Check sheet for the modelled part. Datum: model origin and axes. Units: mm. Face numbers are marked on the shaded views. A direction names the side the tool comes from. Give positions to 0.01 mm unless a question says otherwise; leave off trailing zeros. Order: outer loops, then holes, each group sorted by start corner. A loop starts at its lowest first (then second) coordinate and runs counter-clockwise, first axis right, second up.
from build123d import *

# Parameters (mm, degrees)
SKETCH1_W           = 254
SKETCH1_H           = 63.5
BOSS_EXTRUDE1_DEPTH = 76.2
SHELL1_T            = -3.175
CUT_EXTRUDE1_REACH  = 163.145
SKETCH2_W           = 38.1
SKETCH2_H           = 25.4
SKETCH3_R           = 2.5
CUT_EXTRUDE2_DEPTH  = 162.144934764
SKETCH4_W           = 161.29
SKETCH4_H           = 40.64
CUT_EXTRUDE3_DEPTH  = 152.471127612


with BuildPart() as part:
    # Sketch1 → Boss-Extrude1 (new body)
    with BuildSketch(Plane(origin=(0, 0, 0), x_dir=(1, 0, 0), z_dir=(0, 1, 0))):
        Rectangle(SKETCH1_W, SKETCH1_H)
    extrude(amount=BOSS_EXTRUDE1_DEPTH)

    # Shell1
    shell1_openings = [part.faces().sort_by_distance(p)[0] for p in [
        (0, 0, 0),
    ]]
    offset(amount=SHELL1_T, openings=shell1_openings, kind=Kind.INTERSECTION)

    # Sketch2 → Cut-Extrude1 (cut, up to next)
    with BuildSketch(Plane.XY.offset(31.75), mode=Mode.PRIVATE) as cut_extrude1_sk1:
        with Locations((63.5, 38.1)):
            Rectangle(SKETCH2_W, SKETCH2_H)
    cut_extrude1_tool1 = extrude(cut_extrude1_sk1.sketch, amount=-CUT_EXTRUDE1_REACH, mode=Mode.PRIVATE) & part.part
    # Sketch2 → Cut-Extrude1 (cut, up to next)
    with BuildSketch(Plane.XY.offset(31.75), mode=Mode.PRIVATE) as cut_extrude1_sk2:
        with Locations((-63.5, 38.1)):
            Rectangle(SKETCH2_W, SKETCH2_H)
    cut_extrude1_tool2 = extrude(cut_extrude1_sk2.sketch, amount=-CUT_EXTRUDE1_REACH, mode=Mode.PRIVATE) & part.part
    add(cut_extrude1_tool1.solids().sort_by_distance((63.5, 38.1, 31.75))[0], mode=Mode.SUBTRACT)
    add(cut_extrude1_tool2.solids().sort_by_distance((-63.5, 38.1, 31.75))[0], mode=Mode.SUBTRACT)

    # Sketch3 → Cut-Extrude2 (cut, through all)
    with BuildSketch(Plane(origin=(0, 0, -31.75), x_dir=(-1, 0, 0), z_dir=(0, 0, -1))):
        with Locations((0, 69.85)):
            Circle(SKETCH3_R)
    extrude(amount=-CUT_EXTRUDE2_DEPTH, mode=Mode.SUBTRACT)

    # Sketch4 → Cut-Extrude3 (cut, through all)
    with BuildSketch(Plane(origin=(0, 76.2, 0), x_dir=(1, 0, 0), z_dir=(0, 1, 0))):
        Rectangle(SKETCH4_W, SKETCH4_H)
    extrude(amount=-CUT_EXTRUDE3_DEPTH, mode=Mode.SUBTRACT)


solid = part.part
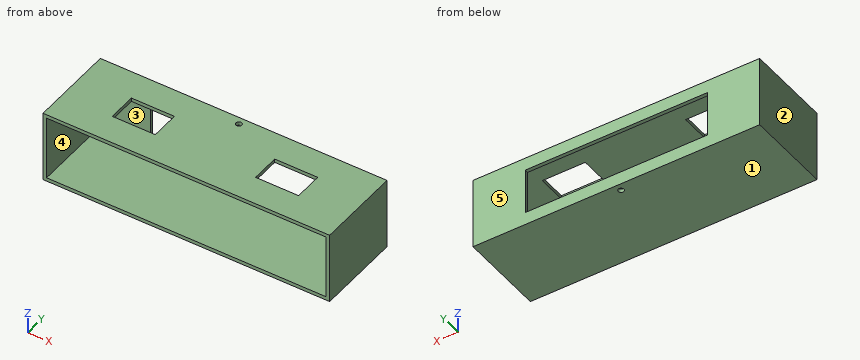
1) Section check B-B, the plane y = 69.85. Record the cut outline in (x, z) (3 decimals), then the cut area to 3 significant figures.
Recorded:
outline: (-127, -31.75) - (-2.5, -31.75) - (-2.5, -28.575) - (-123.825, -28.575) - (-123.825, 28.575) - (-2.5, 28.575) - (-2.5, 31.75) - (-127, 31.75) - close; (2.5, -31.75) - (127, -31.75) - (127, 31.75) - (2.5, 31.75) - (2.5, 28.575) - (123.825, 28.575) - (123.825, -28.575) - (2.5, -28.575) - close
area: 1,940 mm2
2) Draft check along X on the marked faces 1, 2 and 3. Enter one of: +X half, -X half, draft (parallel to the pull), parting line (faces both ways), or undercut.
Recorded:
face 1: draft
face 2: -X half
face 3: undercut
3) Material ranges on L1, parallel to Y at x = 0, z = -30.95; L2, parallel to Z at x = -28, y = 20 (3 decimals); L3, parallel to X at y = 34, z = 22.5 (3 decimals), recorded low to high.
Recorded:
L1: y = 0 to 67.35, 72.35 to 76.2
L2: z = -31.75 to -28.575, 28.575 to 31.75
L3: x = -127 to -123.825, 123.825 to 127
4) Set-up check for the marked faces 4 and 5: record each of +Z, -Z, +X, -X, +Y, -Y from which the full face is reachable in a straight line by a thin tool's end or side.
Recorded:
face 4: -Y
face 5: +Z, -Z, +X, -X, +Y
5) Section check A-A, the plane x = 58. Record the cut outline in (y, z) (3 decimals), then the cut area to 3 significant figures.
Recorded:
outline: (0, -31.75) - (76.2, -31.75) - (76.2, -20.32) - (73.025, -20.32) - (73.025, -28.575) - (0, -28.575) - close; (0, 28.575) - (25.4, 28.575) - (25.4, 31.75) - (0, 31.75) - close; (50.8, 28.575) - (73.025, 28.575) - (73.025, 20.32) - (76.2, 20.32) - (76.2, 31.75) - (50.8, 31.75) - close
area: 456 mm2
6) Section check C-C, the plane x = 7.5. Record the cut outline in (y, z) (3 decimals).
Recorded:
outline: (0, -31.75) - (76.2, -31.75) - (76.2, -20.32) - (73.025, -20.32) - (73.025, -28.575) - (0, -28.575) - close; (0, 28.575) - (73.025, 28.575) - (73.025, 20.32) - (76.2, 20.32) - (76.2, 31.75) - (0, 31.75) - close
7) Section check D-D, the plane y = 8. Record the cut outline in (x, z) (3 decimals).
Recorded:
outline: (-127, -31.75) - (127, -31.75) - (127, 31.75) - (-127, 31.75) - close; hole (-123.825, -28.575) - (123.825, -28.575) - (123.825, 28.575) - (-123.825, 28.575) - close
